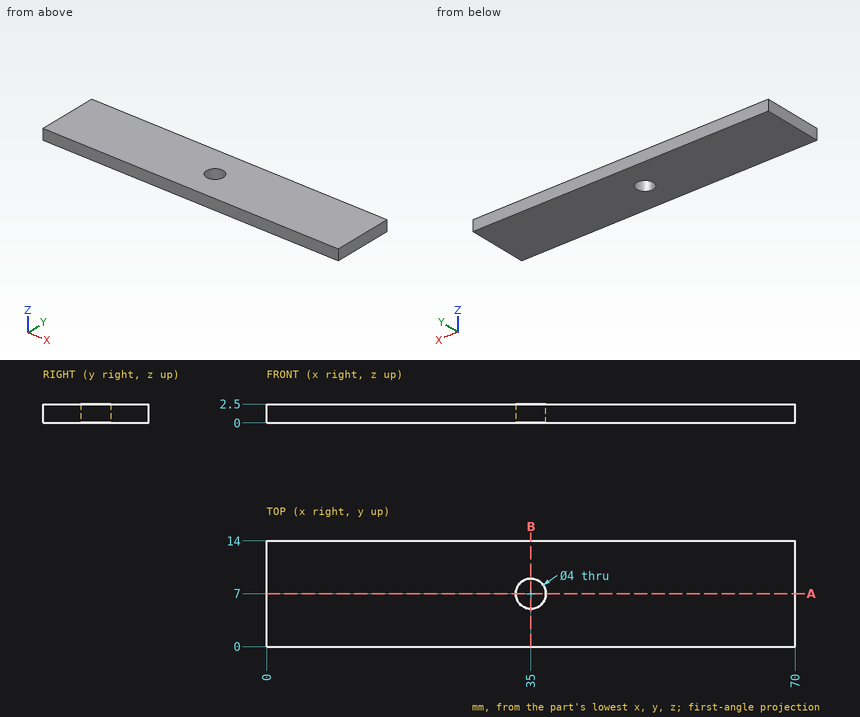
Geometry: see drawing. Coordinates: mm, zero at the bounding-box minimum. Give positions to 0.01 mm unless a question says otherwise; leave off trailing zeros. Loops run counter-clockwise (first coordinate to the right, second up) from the corner with the lowest first, then second, coordinate; pieces in that order, holes last. Notation, with made-up numbers: (11, -18) -> (21, -18) arc R14 ccw to (21, 9) -> close; hole circle Ø7 at (85, -2.75). An arc over 180 degrees is marked (long way). Answer as a JSON object with one key per item and string values. Group by question number.
Item 1: Line query: probe 1 along Y at (x, z) = (35, 1.85); probe 2 along X at (y, z) = (7, 1.95); probe 3 along X at (y, z) = (7.5, 0.95). Output: solid intervals per line, ascending.
Item 2: Pin query (flat end, axial travel): P1, Ø3.5, axis at x = 35, y = 7, coming from the -Z side. Return the tip coordinate at first contact, or that it passes through.
Item 3: Cut plane A-A, the plane y = 7. Return the cut outline in (x, z).
Item 4: Cut plane B-B, the plane x = 35. Return the cut outline in (y, z).
Checks:
{
 "1": {"probe 1": "y = 0 to 5, 9 to 14", "probe 2": "x = 0 to 33, 37 to 70", "probe 3": "x = 0 to 33.06, 36.94 to 70"},
 "2": {"P1": "passes through"},
 "3": {"outline": "(0, 0) -> (33, 0) -> (33, 2.5) -> (0, 2.5) -> close; (37, 0) -> (70, 0) -> (70, 2.5) -> (37, 2.5) -> close"},
 "4": {"outline": "(0, 0) -> (5, 0) -> (5, 2.5) -> (0, 2.5) -> close; (9, 0) -> (14, 0) -> (14, 2.5) -> (9, 2.5) -> close"}
}
